```python
from build123d import *

# Parameters (mm, degrees)
BOSS_EXTRUDE1_DEPTH = 38.1
CHAMFER1_SIZE       = 0.254


with BuildPart() as part:
    # Sketch1 → Boss-Extrude1 (new body, symmetric)
    with BuildSketch(Plane.XY):
        with BuildLine():
            Line((1.905, 2.54), (-1.905, 2.54))
            ThreePointArc((-1.905, 2.54), (0, -3.175), (1.905, 2.54))
        make_face()
    extrude(amount=BOSS_EXTRUDE1_DEPTH, both=True)

    # Chamfer1
    chamfer1_edges = [part.edges().sort_by_distance(p)[0] for p in [
        (0, 2.54, -38.1),
        (0, -3.175, -38.1),
        (0, -3.175, 38.1),
        (0, 2.54, 38.1),
    ]]
    chamfer(chamfer1_edges, length=CHAMFER1_SIZE)


solid = part.part
```
Source: CAD feature listing. Evaluate the final solid. Frame: model axes, mm. Round coordinates to 2 decimals unless told otherwise and drop trailing zeros. Loops run counter-clockwise (first coordinate to the right, second up) from the corner with the lowest first, then second, coordinate; pieces in that order, holes last. Notation, with made-up numbers: M 18,82 L 29,82 A31 cw 29,111 Z; hole C 28,-38 d7. An arc over 180 degrees is marked long. Use a Markdown table: item, result. Add a question column.
1. Contact query for a flat-ended pin moving along its axis: pin 1 (3 mm diameter, centred on y = 2, z = 27, fed in from -X). Output: stop coordinate, or through.
2. Ray query, line 1 along Y through (x, z) = (-1.25, 0.5); line 2 along Z through (x, y) = (0.75, 2.3); line 3 along X through (y, z) = (-1.75, 5.5). Return the intervals inside material, ascending. Write a range as [from, to].
3. Cut plane A-A, the plane z = 7.5. Output: boundary loops of the cut face in (x, y) (3 decimals).
Solution:
| question | item | result |
|---|---|---|
| 1 | pin 1 | stops at x = -3.14 |
| 2 | line 1 | y = [-2.92, 2.54] |
| 2 | line 2 | z = [-38.09, 38.09] |
| 2 | line 3 | x = [-2.65, 2.65] |
| 3 | outline | M -1.905,2.54 A3.175 ccw long 1.905,2.54 Z |
